```python
from build123d import *

# Parameters (mm, degrees)
SKETCH_W        = 29
SKETCH_H        = 38
PAD_DEPTH       = 22
SKETCH001_W     = 25
SKETCH001_H     = 34
POCKET_DEPTH    = 20
SKETCH002_W     = 5.7
SKETCH002_H     = 5.7
PAD001_DEPTH    = 5
SKETCH003_R     = 1.25
POCKET001_DEPTH = 5
FILLET_R        = 2.85
FILLET001_R     = 1
FILLET002_R     = 3


with BuildPart() as part:
    # Sketch → Pad (new body)
    with BuildSketch(Plane.XY):
        Rectangle(SKETCH_W, SKETCH_H)
    extrude(amount=PAD_DEPTH)

    # Sketch001 (on DatumPlane) → Pocket (cut)
    with BuildSketch(Plane.XY.offset(22)):
        Rectangle(SKETCH001_W, SKETCH001_H)
    extrude(amount=-POCKET_DEPTH, mode=Mode.SUBTRACT)

    # Sketch002 (on DatumPlane) → Pad001 (join)
    with BuildSketch(Plane.XY.offset(2)):
        with Locations((-9.65, 14.15)):
            Rectangle(SKETCH002_W, SKETCH002_H)
        with Locations((9.65, 14.15)):
            Rectangle(SKETCH002_W, SKETCH002_H)
        with Locations((9.65, -14.15)):
            Rectangle(SKETCH002_W, SKETCH002_H)
        with Locations((-9.65, -14.15)):
            Rectangle(SKETCH002_W, SKETCH002_H)
    extrude(amount=PAD001_DEPTH)

    # Sketch003 (on DatumPlane) → Pocket001 (cut)
    with BuildSketch(Plane.XY.offset(7)):
        with Locations((-9.65, 14.15)):
            Circle(SKETCH003_R)
        with Locations((9.65, 14.15)):
            Circle(SKETCH003_R)
        with Locations((9.65, -14.15)):
            Circle(SKETCH003_R)
        with Locations((-9.65, -14.15)):
            Circle(SKETCH003_R)
    extrude(amount=-POCKET001_DEPTH, mode=Mode.SUBTRACT)

    # Fillet
    fillet_edges = [part.edges().sort_by_distance(p)[0] for p in [
        (6.8, 11.3, 4.5),
        (-6.8, 11.3, 4.5),
        (-6.8, -11.3, 4.5),
        (6.8, -11.3, 4.5),
    ]]
    fillet(fillet_edges, radius=FILLET_R)

    # Fillet001
    fillet001_edges = [part.edges().sort_by_distance(p)[0] for p in [
        (-12.5, 0, 2),
        (0, 17, 2),
        (12.5, 0, 2),
        (0, -17, 2),
        (-12.5, 17, 14.5),
        (-12.5, -17, 14.5),
        (12.5, 17, 14.5),
        (12.5, -17, 14.5),
    ]]
    fillet(fillet001_edges, radius=FILLET001_R)

    # Fillet002
    fillet002_edges = [part.edges().sort_by_distance(p)[0] for p in [
        (0, 19, 0),
        (14.5, 19, 11),
        (14.5, 0, 0),
        (14.5, -19, 11),
        (0, -19, 0),
        (-14.5, -19, 11),
        (-14.5, 0, 0),
        (-14.5, 19, 11),
    ]]
    fillet(fillet002_edges, radius=FILLET002_R)


solid = part.part
```
The model under review builds one solid part; all positions refer to its coordinate system, in mm. A direction names the side the tool comes from. Round coordinates to 2 decimals unless told otherwise and drop trailing zeros. Write each loop counter-clockwise with the first axis right and the second up, starting at its lowest first coordinate (ties: lowest second). Pieces come first, ordered by that corner, then holes.
(1) Insertion check: pin 1 (0.8 mm diameter, centred on x = -10, y = -14, fed in from +Z); pin 2 (2 mm diameter, centred on x = 9.5, y = 14.5, fed in from +Z). Each pin has a flat end and moves straight along its axis. Give the tip position at first contact, or say it passes through.
(2) Wall thickness on L1, parallel to Y at x = -9.65, z = 5.85; L2, parallel to Y at x = 0.5, z = 8.25; L3, parallel to X at y = -12.5, z = 14.5: over which ranges is each line inside the solid? List them lowest first.
(3) We need section C-C on y = -2.5. Give the boundary of the cut face in (x, z), and give its area (3 significant figures).
(4) We need section A-A on z = 4.75. Give the boundary of the cut face in (x, y), and give its area (3 significant figures).
(5) We need section D-D on x = -1.75. Give the boundary of the cut face in (y, z).
(6) We need section B-B on z = 8.5. Give the boundary of the cut face in (x, y).
(7) Machinability: for faces 1 (the cylindrical face through (-13.64, 18.1, 12.63)), 2 (the flat face through (-6.8, -16, 4)), which of the approach directions +Z, -Z, +X, -X, +Y, -Y give a long, thin tool a straight path to every point of the face, cutting with its end or side? Answer none if there is none.
Findings below:
1. pin 1: stops at z = 2
1. pin 2: stops at z = 7
2. L1: y = -19 to -15.4, -12.9 to -11.3, 11.3 to 12.9, 15.4 to 19
2. L2: y = -19 to -17, 17 to 19
2. L3: x = -14.5 to -12.5, 12.5 to 14.5
3. outline: (-14.5, 3) arc R3 ccw to (-11.5, 0) - (11.5, 0) arc R3 ccw to (14.5, 3) - (14.5, 22) - (12.5, 22) - (12.5, 3) arc R1 cw to (11.5, 2) - (-11.5, 2) arc R1 cw to (-12.5, 3) - (-12.5, 22) - (-14.5, 22) - close
3. area: 135 mm2
4. outline: (-14.5, -16) arc R3 ccw to (-11.5, -19) - (11.5, -19) arc R3 ccw to (14.5, -16) - (14.5, 16) arc R3 ccw to (11.5, 19) - (-11.5, 19) arc R3 ccw to (-14.5, 16) - close; hole (-12.5, -11.3) - (-9.65, -11.3) arc R2.85 cw to (-6.8, -14.15) - (-6.8, -17) - (6.8, -17) - (6.8, -14.15) arc R2.85 cw to (9.65, -11.3) - (12.5, -11.3) - (12.5, 11.3) - (9.65, 11.3) arc R2.85 cw to (6.8, 14.15) - (6.8, 17) - (-6.8, 17) - (-6.8, 14.15) arc R2.85 cw to (-9.65, 11.3) - (-12.5, 11.3) - close; hole circle Ø2.5 at (-9.65, -14.15); hole circle Ø2.5 at (-9.65, 14.15); hole circle Ø2.5 at (9.65, -14.15); hole circle Ø2.5 at (9.65, 14.15)
4. area: 348 mm2
5. outline: (-19, 3) arc R3 ccw to (-16, 0) - (16, 0) arc R3 ccw to (19, 3) - (19, 22) - (17, 22) - (17, 3) arc R1 cw to (16, 2) - (-16, 2) arc R1 cw to (-17, 3) - (-17, 22) - (-19, 22) - close
6. outline: (-14.5, -16) arc R3 ccw to (-11.5, -19) - (11.5, -19) arc R3 ccw to (14.5, -16) - (14.5, 16) arc R3 ccw to (11.5, 19) - (-11.5, 19) arc R3 ccw to (-14.5, 16) - close; hole (-12.5, -16) arc R1 ccw to (-11.5, -17) - (11.5, -17) arc R1 ccw to (12.5, -16) - (12.5, 16) arc R1 ccw to (11.5, 17) - (-11.5, 17) arc R1 ccw to (-12.5, 16) - close
7. face 1: +Z, -Z, -X, +Y
7. face 2: +Z
